Check sheet for the modelled part. Datum: model origin and axes. Units: mm. A direction names the side the tool comes from. Coordinates: 2 decimals unless noted, no trailing zeros. Loops run counter-clockwise (first coordinate to the right, second up) from the corner with the lowest first, then second, coordinate; pieces in that order, holes last. Notation, with made-up numbers: (-33.75, 68) -> (-28.75, 68) arc R15 ccw to (-28.75, 92) -> close; hole circle Ø6 at (58.5, 44). An arc over 180 degrees is marked (long way). Use one line per item in the form item = value.
from build123d import *

# Parameters (mm, degrees)
ESQUISSE1_W        = 5
ESQUISSE1_H        = 3
BOSS_EXTRU_1_DEPTH = 3


with BuildPart() as part:
    # Esquisse1 → Boss.-Extru.1 (new body)
    with BuildSketch(Plane.XY):
        Polygon((-20, -5), (-20, 0), (-15, 0), (-15, -5), (-10, -5), (-10, 0), (-5, 0), (-5, -5), (0, -5), (0, 15.5), (-35, 15.5), (-35, -5), (-30, -5), (-30, 0), (-25, 0), (-25, -5), align=None)
        with Locations((-7.5, 9)):
            Rectangle(ESQUISSE1_W, ESQUISSE1_H, mode=Mode.SUBTRACT)
        with Locations((-17.5, 9)):
            Rectangle(ESQUISSE1_W, ESQUISSE1_H, mode=Mode.SUBTRACT)
        with Locations((-27.5, 9)):
            Rectangle(ESQUISSE1_W, ESQUISSE1_H, mode=Mode.SUBTRACT)
        with Locations((-7.5, 4.5)):
            Rectangle(ESQUISSE1_W, ESQUISSE1_H, mode=Mode.SUBTRACT)
        with Locations((-17.5, 4.5)):
            Rectangle(ESQUISSE1_W, ESQUISSE1_H, mode=Mode.SUBTRACT)
        with Locations((-27.5, 4.5)):
            Rectangle(ESQUISSE1_W, ESQUISSE1_H, mode=Mode.SUBTRACT)
    extrude(amount=BOSS_EXTRU_1_DEPTH)


solid = part.part
(1) Section check B-B, the plane x = -28. Record the boundary of the cut face in (y, z), plus the area to 3 significant figures.
Established:
outline = (0, 0) -> (3, 0) -> (3, 3) -> (0, 3) -> close; (6, 0) -> (7.5, 0) -> (7.5, 3) -> (6, 3) -> close; (10.5, 0) -> (15.5, 0) -> (15.5, 3) -> (10.5, 3) -> close
area = 28.5 mm²
(2) Section check A-A, the plane y = 9. Record the boundary of the cut face in (x, z), plus the area to 3 significant figures.
Established:
outline = (-35, 0) -> (-30, 0) -> (-30, 3) -> (-35, 3) -> close; (-25, 0) -> (-20, 0) -> (-20, 3) -> (-25, 3) -> close; (-15, 0) -> (-10, 0) -> (-10, 3) -> (-15, 3) -> close; (-5, 0) -> (0, 0) -> (0, 3) -> (-5, 3) -> close
area = 60.0 mm²
(3) Scan lines: line 1 along X through (y, z) = (-1, 0.55); line 2 along Y through (x, z) = (-8, 1.65). Record each from-to range of solid material in increasing order.
Established:
line_1 = -35 to -30, -25 to -20, -15 to -10, -5 to 0
line_2 = 0 to 3, 6 to 7.5, 10.5 to 15.5
(4) Mould release check, pull along Y, two halves, no side actions. Record for faces 4 (the flat face through (-10, 9, 1)), 5 (the flat face through (-17, 15.5, 1)), 6 (the flat face through (-20, -3, 1)): +Y half, -Y half, draft (parallel to the pull), parting line (faces both ways), or undercut.
Established:
face_4 = undercut
face_5 = +Y half
face_6 = draft
(5) Section check C-C, the plane z = 2.5. Give the number of separate pieces and of enclosed holes in the cut face, plus the area to 4 significant figures.
Established:
separate_pieces = 1
enclosed_holes = 6
area = 552.5 mm²
(6) Go/stop test with a flat-tipped pin: P1, Ø0.9, axis at x = -6.5, z = 2, coming from the -Y side. Record where the tip stops, or that it passes through.
Established:
P1 = 0
(7) Tool access check on faces 1 (the flat face through (-15, -2, 1)), 2 (the flat face through (-23, -5, 1)), 3 (the flat face through (-20, 9, 1)). Record the directions out of +Z, -Z, +X, -X, +Y, -Y that give a thin tool (end or side, any length) a straight path to the whole face; none if there is none.
Established:
face_1 = +Z, -Z, -Y
face_2 = +Z, -Z, +X, -X, -Y
face_3 = +Z, -Z
